Autodesk Inventor part; units mm, degrees
ref_plane "YZ Plane" through (0, 0, 0) normal (1, 0, 0) x (0, 1, 0)
ref_plane "XZ Plane" through (0, 0, 0) normal (0, 1, 0) x (-1, 0, 0)
ref_plane "XY Plane" through (0, 0, 0) normal (0, 0, 1) x (1, 0, 0)
sketch "スケッチ1" plane through (0, 0, 0) normal (0, 0, 1) x (1, 0, 0)
  circle A0 centre (0, 0) radius 2.5
  line L0 (-15, 15) -> (15, 15)
  line L1 (15, 15) -> (15, -15)
  line L2 (15, -15) -> (-15, -15)
  line L3 (-15, -15) -> (-15, 15)
  line L4 (-15, 15) -> (15, -15) construction
  line L5 (15, 15) -> (-15, -15) construction
  line L6 (-3, 17.5) -> (3, 17.5)
  line L7 (3, 17.5) -> (3, 12.5)
  line L8 (3, 12.5) -> (-3, 12.5) construction
  line L9 (-3, 12.5) -> (-3, 17.5)
  line L10 (-3, 17.5) -> (3, 12.5) construction
  line L11 (3, 17.5) -> (-3, 12.5) construction
  line L12 (4.5, -4.5) -> (-4.5, -4.5)
  line L13 (-4.5, -4.5) -> (-4.5, 4.5)
  line L14 (-4.5, 4.5) -> (4.5, 4.5)
  line L15 (4.5, 4.5) -> (4.5, -4.5)
  line L16 (4.5, -4.5) -> (-4.5, 4.5) construction
  line L17 (-4.5, -4.5) -> (4.5, 4.5) construction
  line L18 (-7, 7) -> (7, 7)
  line L19 (7, 7) -> (7, -7)
  line L20 (7, -7) -> (-7, -7)
  line L21 (-7, -7) -> (-7, 7)
  line L22 (-7, 7) -> (7, -7) construction
  line L23 (7, 7) -> (-7, -7) construction
  line L24 (-7, 7) -> (-3, 7)
  line L25 (-3, 7) -> (-3, 3)
  line L26 (-3, 3) -> (-7, 3)
  line L27 (-7, 3) -> (-7, 7)
  line L28 (-7, -3) -> (-3, -3)
  line L29 (-3, -3) -> (-3, -7)
  line L30 (3, -7) -> (3, -3)
  line L31 (3, -3) -> (7, -3)
  line L32 (7, 3) -> (3, 3)
  line L33 (3, 3) -> (3, 7)
  line L34 (-15, 15) -> (-5, 15)
  line L35 (-5, 15) -> (-5, 5)
  line L36 (-5, 5) -> (-15, 5)
  line L37 (-15, 5) -> (-15, 15)
  line L38 (-15, -5) -> (-5, -5)
  line L39 (-5, -5) -> (-5, -15)
  line L40 (5, -15) -> (5, -5)
  line L41 (5, -5) -> (15, -5)
  line L42 (15, 5) -> (5, 5)
  line L43 (5, 5) -> (5, 15)
  line L44 (-3, 12.5) -> (-5, 12.5)
  line L45 (3, 12.5) -> (5, 12.5)
  line L46 (-12.5, -3) -> (-12.5, -5)
  line L47 (-12.5, -3) -> (-17.5, -3)
  line L48 (-17.5, 3) -> (-12.5, 3)
  line L49 (-12.5, 3) -> (-12.5, 5)
  line L50 (3, -12.5) -> (5, -12.5)
  line L51 (3, -12.5) -> (3, -17.5)
  line L52 (-3, -17.5) -> (-3, -12.5)
  line L53 (-3, -12.5) -> (-5, -12.5)
  line L54 (12.5, 3) -> (12.5, 5)
  line L55 (12.5, 3) -> (17.5, 3)
  line L56 (17.5, -3) -> (12.5, -3)
  line L57 (12.5, -3) -> (12.5, -5)
  line L58 (-13.5, 13.5) -> (-6.5, 13.5)
  line L59 (-6.5, 13.5) -> (-6.5, 6.5)
  line L60 (-6.5, 6.5) -> (-13.5, 6.5)
  line L61 (-13.5, 6.5) -> (-13.5, 13.5)
  point P0 (0, 15)
  point P1 (-7, 5)
  point P2 (-4.5, 3)
  point P3 (-4.5, -3)
  point P4 (-7, -5)
  point P5 (-15, -3)
  point P6 (-3, -15)
  point P7 (-5, -7)
  point P8 (-3, -4.5)
  point P9 (3, -4.5)
  point P10 (5, -7)
  point P11 (3, -15)
  point P12 (15, -3)
  point P13 (7, -5)
  point P14 (4.5, -3)
  point P15 (4.5, 3)
  point P16 (7, 5)
  point P17 (15, 3)
  point P18 (3, 15)
  point P19 (5, 7)
  point P20 (3, 4.5)
  point P21 (-3, 4.5)
  point P22 (-5, 7)
  point P23 (-3, 15)
  point P24 (-15, 3)
  point P25 (-7, 6.5)
  point P26 (-6.5, 7)
  dimension "d0" = 5
  dimension "d1" = 30
  dimension "d2" = 30
  dimension "d3" = 6
  dimension "d4" = 5
  dimension "d5" = 9
  dimension "d6" = 9
  dimension "d7" = 14
  dimension "d8" = 14
  dimension "d9" = 4
  dimension "d10" = 4
  dimension "d13" = 360
  dimension "d15" = 10
  dimension "d16" = 10
  dimension "d19" = 360
  dimension "d23" = 360
  dimension "d27" = 1.5
  dimension "d28" = 7
extrude "押し出し1" add sketch "スケッチ1" along normal blind 260 contours L0 L35 L18 L59 L58 L61 L60 L21 L36 L3 | L0 L9 L44 L35 | L36 L49 L48 L3 | L0 L43 L45 L7 | L35 L36 L21 L60 L59 L18 | L18 L25 L14 L13 L26 L21 L36 L35 | L47 L46 L38 L3 | L0 L1 L42 L19 L18 L43 | L59 L60 L21 L18 | L18 L21 L60 L61 L58 L59 | L38 L21 L20 L39 L2 L3 | L18 L43 L42 L19 L32 L15 L14 L33 | L25 L26 L13 L14 | L14 L33 L32 L15 L31 L30 L12 L29 L28 L13 L26 L25 | L28 L13 L12 L29 L20 L39 L38 L21 | L1 L55 L54 L42 | L18 L19 L42 L43 | L14 L15 L32 L33 | L39 L53 L52 L2 | L38 L39 L20 L21 | L28 L29 L12 L13 | L1 L41 L57 L56 | L51 L50 L40 L2 | L1 L2 L40 L20 L19 L41 | L31 L19 L41 L40 L20 L30 L12 L15 | L15 L12 L30 L31 | L19 L20 L40 L41
extrude "押し出し2" cut sketch "スケッチ1" along normal blind 260 contours L18 L21 L60 L61 L58 L59
pattern_circular "円形状パターン1" count 4 over 360 about axis through (0, 0, 0) along (0, 0, 1) of "押し出し2"
properties part number "baicPart" material "アルミニウム"
Model file for the job. Use its own axes, mm. A direction names the side the tool comes from. Round coordinates to 2 decimals unless told otherwise and drop trailing zeros. Order: outer loops, then holes, each group sorted by start corner. A loop starts at its lowest first (then second) coordinate and runs counter-clockwise, first axis right, second up.
(1) Pull direction Y, two halves, no side cores. Call faces 1 (the face through (-15, 9, 128)), 2 (the face through (-10, 5, 128)), 3 (the face through (0, 4.5, 128)), 4 (the face through (10, -6.5, 128)): released by +Y, released by -Y, zero draft, split by the parting line, or undercut.
(2) 3-axis set-ups, long thin cutter, end or side, ignore diameter. For faces 5 (the face through (4.5, 0, 128)), 6 (the face through (-4.5, 0, 128)), 7 (the face through (-10, 13.5, 128)): which of +Z, -Z, +X, -X, +Y, -Y reach the whole face in a straight line?
(3) Band-saw the part on A-A (y = 0). List the corners of the cut face in (x, z).
(4) Drill centre lines: line 1 (Y direction, x = -7.5, z = 134); line 2 (Y direction, x = 4, z = 118). Where is each one in solid material? Low to high.
(5) Band-saw the part on C-C (z = 158). Give the number of separate pieces and of enclosed holes in the cut face, then the cut area to 3 significant figures.
(6) Pin check, flat tip, straight feed: pin 1 (2 mm diameter, centred on x = 1.5, z = 118, fed in from +Y). Stop position of the tip, or through.
Verdict:
1. face 1: zero draft
1. face 2: undercut
1. face 3: released by +Y
1. face 4: undercut
2. face 5: +Z, -Z, +X
2. face 6: +Z, -Z, -X
2. face 7: +Z, -Z
3. outline: (-4.5, 0) - (-2.5, 0) - (-2.5, 260) - (-4.5, 260) - close; (2.5, 0) - (4.5, 0) - (4.5, 260) - (2.5, 260) - close
4. line 1: y = -15 to -13.5, -6.5 to -5, 5 to 6.5, 13.5 to 15
4. line 2: y = -15 to -12.5, -7 to 7, 12.5 to 15
5. separate pieces: 1
5. enclosed holes: 5
5. area: 345 mm2
6. pin 1: stops at y = 4.5
